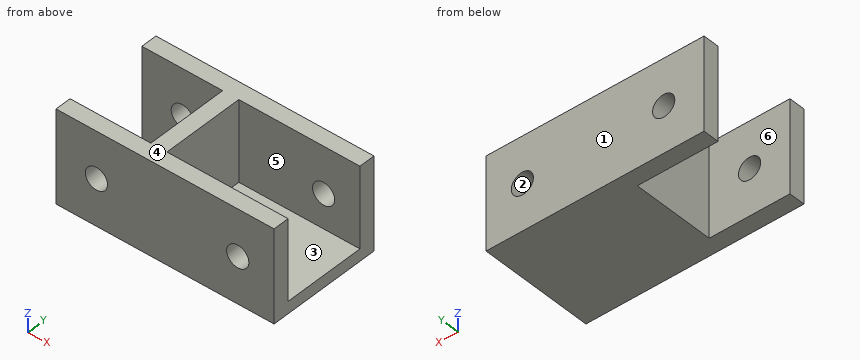
from build123d import *

# Parameters (mm, degrees)
PAD043_DEPTH            = 11.5
SKETCH069_W             = 10.25
SKETCH069_H             = 30
PAD044_DEPTH            = 3
SKETCH070_R             = 2.75
POCKET020_DEPTH         = 5
BODY033_PLACEMENT_ANGLE = 90


with BuildPart() as part:
    # Sketch068 → Pad043 (new body, symmetric)
    with BuildSketch(Plane.XY):
        Polygon((0, 0), (10.25, 0), (10.25, 20), (14.25, 20), (14.25, -34), (10.25, -34), (10.25, -4), (0, -4), align=None)
    pad043 = extrude(amount=PAD043_DEPTH, both=True)

    # Sketch069 (on Face9 of Pad043) → Pad044 (join)
    with BuildSketch(Plane(origin=(0, 0, -11.5), x_dir=(1, 0, 0), z_dir=(0, 0, -1))):
        with Locations((5.125, 19)):
            Rectangle(SKETCH069_W, SKETCH069_H)
    pad044 = extrude(amount=-PAD044_DEPTH)

    # Sketch070 (on Face9 of Pad044) → Pocket020 (cut)
    with BuildSketch(Plane.YZ.offset(14.25)):
        with Locations((-25, 0)):
            Circle(SKETCH070_R)
        with Locations((10, 0)):
            Circle(SKETCH070_R)
    pocket020 = extrude(amount=-POCKET020_DEPTH, mode=Mode.SUBTRACT)

    # Mirrored019: Pad043, Pad044, Pocket020 across Sketch068 V_Axis
    add(pad043.mirror(Plane(origin=(0, 0, 0), x_dir=(0, 0, 1), z_dir=(1, 0, 0))))
    add(pad044.mirror(Plane(origin=(0, 0, 0), x_dir=(0, 0, 1), z_dir=(1, 0, 0))))
    add(pocket020.mirror(Plane(origin=(0, 0, 0), x_dir=(0, 0, 1), z_dir=(1, 0, 0))), mode=Mode.SUBTRACT)


with BuildPart() as part_1:
    # Body033 placement: moved
    add(part.part.moved(Location((-140, 0, 0))).rotate(Axis((-140, 0, 0), (0, 0, 1)), BODY033_PLACEMENT_ANGLE))


solid = part_1.part
CAD build for the part. Positions are in the model's coordinates, mm. Face numbers are marked on the shaded views. A direction names the side the tool comes from. Coordinates: 2 decimals unless noted, no trailing zeros. Write each loop counter-clockwise with the first axis right and the second up, starting at its lowest first coordinate (ties: lowest second). Pieces come first, ordered by that corner, then holes. Notation, with made-up numbers: M 37.25,-31.75 L 61.25,-31.75 A30 cw 61.25,-9.75 Z; hole C -22,60.25 d11. An arc over 180 degrees is marked long. Return JSON: item names as keys, results as strings.
Item 1: Two-plate mould, pull along Z, no slides. Class the marked faces 1, 2 and 3: +Z half, -Z half, draft (parallel to the pull), parting line (faces both ways), or undercut.
Findings below:
{"face 1": "draft", "face 2": "undercut", "face 3": "+Z half"}
Item 2: Drop flat-ended pins along their axis: pin 1 Ø12 at (x, y) = (-152, -1.5) entering from +Z; pin 2 Ø3 at (x, y) = (-119, -6) entering from +Z; pin 3 Ø6 at (y, z) = (-6.5, 9) entering from +X; pin 4 Ø1 at (y, z) = (9, 9) entering from -X. Give the stop position or say it passes through.
Findings below:
{"pin 1": "passes through", "pin 2": "stops at z = -8.5", "pin 3": "stops at x = -136", "pin 4": "stops at x = -140"}
Item 3: Probe line 1 (X direction, y = -11.65, z = 0); line 2 (Y direction, x = -147.5, z = -2.25). List the from-to ranges inside material, lowest first. Write a range as from..to.
Findings below:
{"line 1": "x = -160..-152.75, -147.25..-117.75, -112.25..-106", "line 2": "y = -14.25..-10.25, 10.25..14.25"}
Item 4: Slice it at C-C, the plane y = 12.5. Write the cut outline in (x, z).
Findings below:
{"outline": "M -160,-11.5 L -106,-11.5 L -106,11.5 L -160,11.5 Z; hole C -150,0 d5.5; hole C -115,0 d5.5"}
Item 5: Slice it at D-D, the plane z = -5.5. Write the cut outline in (x, y), and give its area (3 significant figures).
Findings below:
{"outline": "M -160,-14.25 L -106,-14.25 L -106,-10.25 L -136,-10.25 L -136,10.25 L -106,10.25 L -106,14.25 L -160,14.25 L -160,10.25 L -140,10.25 L -140,-10.25 L -160,-10.25 Z", "area": "514 mm2"}
Item 6: Slice it at A-A, the plane x = -115. Write the cut outline in (y, z), and give its area (4 significant figures).
Findings below:
{"outline": "M -14.25,-11.5 L 14.25,-11.5 L 14.25,-2.75 L 10.25,-2.75 L 10.25,-8.5 L -10.25,-8.5 L -10.25,-2.75 L -14.25,-2.75 Z; M -14.25,2.75 L -10.25,2.75 L -10.25,11.5 L -14.25,11.5 Z; M 10.25,2.75 L 14.25,2.75 L 14.25,11.5 L 10.25,11.5 Z", "area": "201.5 mm2"}
Item 7: Slice it at B-B, the plane x = -141. Write the cut outline in (y, z), and give its area (3 significant figures).
Findings below:
{"outline": "M -14.25,-11.5 L -10.25,-11.5 L -10.25,11.5 L -14.25,11.5 Z; M 10.25,-11.5 L 14.25,-11.5 L 14.25,11.5 L 10.25,11.5 Z", "area": "184 mm2"}
Item 8: Which spindle directions (+Z, -Z, +X, -X, +Y, -Y) get a long thin tool onto all of the face, cutting with end or side? Do the marked faces 4, 5 and 6. Say none if no direction does.
Findings below:
{"face 4": "+Z, +X, -X, +Y, -Y", "face 5": "+Z, +X", "face 6": "+Z, -Z, -X"}
